from build123d import *

# Parameters (mm, degrees)
F0_W     = 66
F0_H     = 40
F1_DEPTH = 2
F2_DEPTH = 2
F3_W     = 2
F3_H     = 40
F4_DEPTH = 16
F5_DEPTH = 2
F6_DEPTH = 2
F7_DEPTH = 4
F8_DEPTH = 2


with BuildPart() as f1:
    # F0 (on Top) → F1 (new body)
    with BuildSketch(Plane.XY):
        Rectangle(F0_W, F0_H)
    extrude(amount=F1_DEPTH)

    # F0 (on Top) → F2 (join)
    with BuildSketch(Plane.XY):
        Rectangle(F0_W, F0_H)
    extrude(amount=F2_DEPTH)

    # F3 (on face) → F4 (join)
    with BuildSketch(Plane.XY.offset(2)):
        with Locations((-32, 0)):
            Rectangle(F3_W, F3_H)
        with Locations((32, 0)):
            Rectangle(F3_W, F3_H)
    extrude(amount=F4_DEPTH)

    # F5 (add): a face of the model
    f5_faces = [f1.faces().sort_by_distance(p)[0] for p in [
        (33, 0, 9),
    ]]
    extrude(f5_faces, amount=F5_DEPTH)

    # F6 (add): a face of the model
    f6_faces = [f1.faces().sort_by_distance(p)[0] for p in [
        (-33, 0, 9),
    ]]
    extrude(f6_faces, amount=F6_DEPTH)

    # F7 (add): a face of the model
    f7_faces = [f1.faces().sort_by_distance(p)[0] for p in [
        (0, 0, 0),
    ]]
    extrude(f7_faces, amount=F7_DEPTH)

    # F8 (add): a face of the model
    f8_faces = [f1.faces().sort_by_distance(p)[0] for p in [
        (0, 0, -4),
    ]]
    extrude(f8_faces, amount=F8_DEPTH)


solid = f1.part
Model file for the job. Use its own axes, mm. A direction names the side the tool comes from. Give positions to 0.01 mm unless a question says otherwise; leave off trailing zeros. Loops run counter-clockwise (first coordinate to the right, second up) from the corner with the lowest first, then second, coordinate; pieces in that order, holes last. Notation, with made-up numbers: (39.25, -30.75) - (87.25, -30.75) arc R29 ccw to (87.25, 0.25) - close; hole circle Ø6 at (19.5, -20). An arc over 180 degrees is marked (long way). Use one line per item in the form item = value.
(1) Cut at A-A (z = 3). Give the cut face in (x, y), then the cut area to 3 significant figures.
Determined:
outline = (-35, -20) - (-31, -20) - (-31, 20) - (-35, 20) - close; (31, -20) - (35, -20) - (35, 20) - (31, 20) - close
area = 320 mm^2
(2) Drill centre lines: L1, parallel to X at y = -12.5, z = 13; L2, parallel to Z at x = -22.5, y = 1.5. Where is each one in solid material? Low to high.
Determined:
L1 = -35 to -31, 31 to 35
L2 = -6 to 2
(3) Pull direction X, two halves, no side cores. Call faces 1 (the face through (35, 0, 6)), 2 (the face through (0, 0, -6)), 3 (the face through (31, 0, 10)): pulls with the +X half, pulls with the -X half, needs draft (parallel to the pull), parting line crosses it, or undercut.
Determined:
face_1 = pulls with the +X half
face_2 = needs draft
face_3 = undercut
(4) Cut at B-B (y = 10). Give the cut face in (x, z).
Determined:
outline = (-35, -6) - (35, -6) - (35, 18) - (31, 18) - (31, 2) - (-31, 2) - (-31, 18) - (-35, 18) - close
(5) 3-axis set-ups, long thin cutter, end or side, ignore diameter. For faces 4 (the face through (0, 0, 2)), 5 (the face through (-33, 0, 18)): which of +Z, -Z, +X, -X, +Y, -Y reach the whole face in a straight line?
Determined:
face_4 = +Z, +Y, -Y
face_5 = +Z, +X, -X, +Y, -Y
(6) Drop a flat-ended pin along its axis: P1, Ø5, axis at x = 18.5, y = 13, coming from the +Z side. Give the stop position or say it passes through.
Determined:
P1 = 2
(7) Cut at C-C (x = 14.5). Give the cut face in (y, z).
Determined:
outline = (-20, -6) - (20, -6) - (20, 2) - (-20, 2) - close
